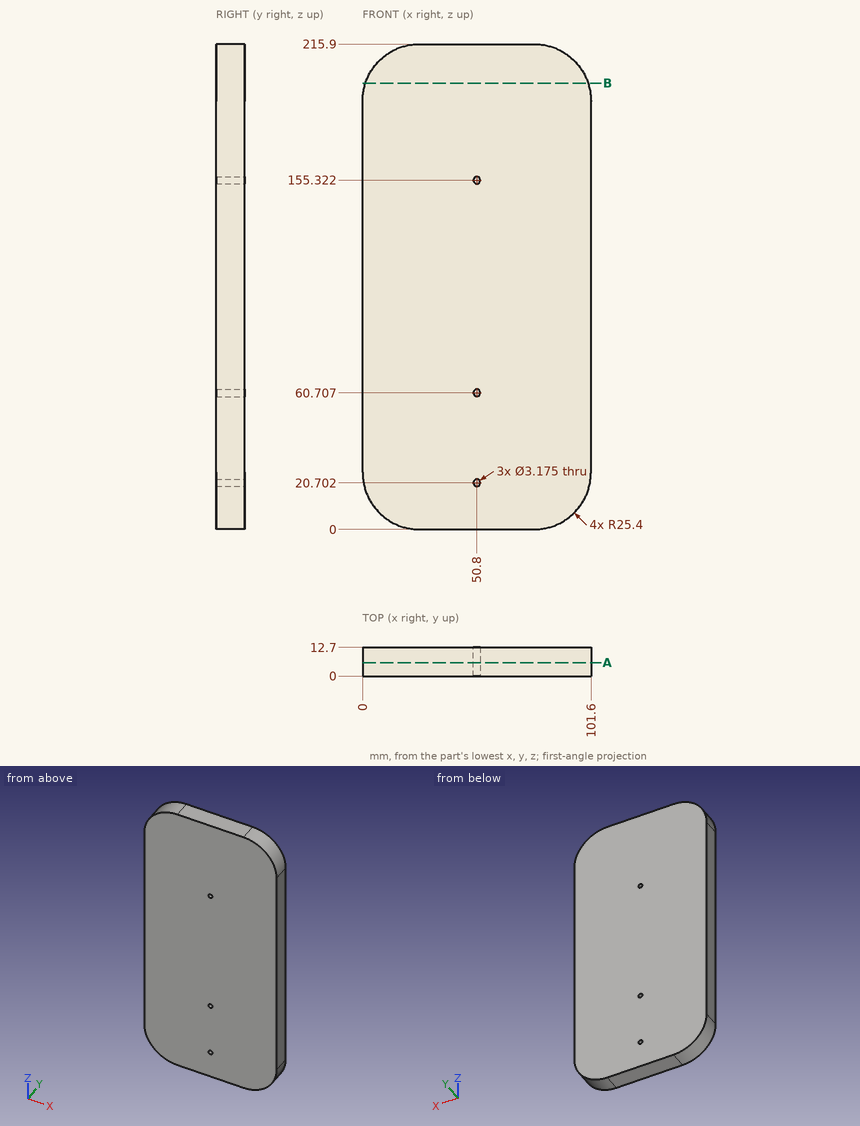
Answer from the drawing. Dimensions are ordinates in mm from the lowest x, y and z of the part. Round coordinates to 2 decimals unless told otherwise and drop trailing zeros. Loops run counter-clockwise (first coordinate to the right, second up) from the corner with the lowest first, then second, coordinate; pieces in that order, holes last. Notation, with made-up numbers: (66.5, 44) - (111.5, 44) arc R22 ccw to (111.5, 66) - close; hole circle Ø1 at (9, -21.5). An arc over 180 degrees is marked (long way). One line per item, written item: value.
Q1. Find section B-B on z = 198.5. Give the vertices of the cut face in (x, y), and give its area (3 significant figures).
Check values:
outline: (1.29, 0) - (100.31, 0) - (100.31, 12.7) - (1.29, 12.7) - close
area: 1,260 mm2
Q2. This flat-tipped pin is pushed along its axis until it touches: pin 1 Ø6 at (y, z) = (8.5, 86.5) entering from -X. Where does it stop, or does it pass through?
Check values:
pin 1: x = 0
Q3. Straight lines are drawn through the part: probe 1 along Z at (x, y) = (50.8, 10) (1 decimal); probe 2 along X at (y, z) = (5, 61); probe 3 along X at (y, z) = (7.5, 191) (1 decimal). For each, find the intervals that lie inside material, in ascending order.
Check values:
probe 1: 0 to 19.1, 22.3 to 59.1, 62.3 to 153.7, 156.9 to 215.9
probe 2: 0 to 49.24, 52.36 to 101.6
probe 3: 0 to 101.6
Q4. Find section A-A on y = 6. Give the vertices of the cut face in (x, z) (1 decimal).
Check values:
outline: (0, 25.4) arc R25.4 ccw to (25.4, 0) - (76.2, 0) arc R25.4 ccw to (101.6, 25.4) - (101.6, 190.5) arc R25.4 ccw to (76.2, 215.9) - (25.4, 215.9) arc R25.4 ccw to (0, 190.5) - close; hole circle Ø3.2 at (50.8, 20.7); hole circle Ø3.2 at (50.8, 60.7); hole circle Ø3.2 at (50.8, 155.3)
